```python
from build123d import *

# Parameters (mm, degrees)
SKETCH1_W           = 70
SKETCH1_H           = 40
BOSS_EXTRUDE1_DEPTH = 6.35
SKETCH2_R           = 12.5
SKETCH2_R_2         = 2
CUT_EXTRUDE1_DEPTH  = 81.872260386


with BuildPart() as part:
    # Sketch1 → Boss-Extrude1 (new body)
    with BuildSketch(Plane(origin=(0, 0, 0), x_dir=(1, 0, 0), z_dir=(0, 1, 0))):
        with Locations((35, 20)):
            Rectangle(SKETCH1_W, SKETCH1_H)
    extrude(amount=BOSS_EXTRUDE1_DEPTH)

    # Sketch2 → Cut-Extrude1 (cut, through all)
    with BuildSketch(Plane(origin=(0, 6.35, 0), x_dir=(1, 0, 0), z_dir=(0, 1, 0))):
        with Locations(Location((49.5, 20, 0), (0, 0, 270))):
            Circle(SKETCH2_R)
        with Locations(Location((34, 35.5, 0), (0, 0, 270))):
            Circle(SKETCH2_R_2)
        with Locations(Location((65, 35.5, 0), (0, 0, 270))):
            Circle(SKETCH2_R_2)
        with Locations(Location((65, 4.5, 0), (0, 0, 270))):
            Circle(SKETCH2_R_2)
        with Locations(Location((34, 4.5, 0), (0, 0, 270))):
            Circle(SKETCH2_R_2)
        with BuildLine():
            Line((10, 25), (0, 25))
            Line((0, 25), (0, 15))
            Line((0, 15), (10, 15))
            ThreePointArc((10, 15), (15, 20), (10, 25))
        make_face()
        with BuildLine():
            Line((13, 28), (7, 28))
            ThreePointArc((7, 28), (5, 30), (7, 32))
            Line((7, 32), (13, 32))
            ThreePointArc((13, 32), (15, 30), (13, 28))
        make_face()
        with BuildLine():
            Line((7, 12), (13, 12))
            ThreePointArc((13, 12), (15, 10), (13, 8))
            Line((13, 8), (7, 8))
            ThreePointArc((7, 8), (5, 10), (7, 12))
        make_face()
    extrude(amount=-CUT_EXTRUDE1_DEPTH, mode=Mode.SUBTRACT)


solid = part.part
```
Geometry: final body of the model. Coordinates: model frame, mm. A direction names the side the tool comes from. Round coordinates to 2 decimals unless told otherwise and drop trailing zeros. Write each loop counter-clockwise with the first axis right and the second up, starting at its lowest first coordinate (ties: lowest second). Pieces come first, ordered by that corner, then holes.
Item 1: Section query D-D (z = -22.5). Return loops of the section in (x, y), plus the area to 3 significant figures.
Item 2: Set-up query: faces 5 (the face through (5, 3, -15)), 6 (the face through (35, 6.35, -20)), 7 (the face through (10, 3, -32)). Return all of +Z, -Z, +X, -X, +Y, -Y with unobstructed straight access to the full face (end or side cutting, diameter ignored); none if empty.
Item 3: Pin query (flat end, axial travel): P1, Ø20, axis at x = 49.5, z = -20, coming from the +Y side. Return the tip coordinate at first contact, or that it passes through.
Item 4: Section query B-B (x = 34). Return loops of the section in (y, z).
Item 5: Mould query, pull axis X, two halves, no side actions, for faces 1 (the face through (35, 3, 0)), 2 (the face through (15, 3, -20)), 3 (the face through (15, 3, -30)), 4 (the face through (10, 3, -12)). Classes: +X half, -X half, draft (parallel to the pull), parting line (faces both ways), or undercut.
Item 6: Section query A-A (z = -30). Return loops of the section in (x, y).
Item 7: Section query C-C (y = 4.5). Return loops of the section in (x, z).
Item 8: Material intervals for L1, parallel to X at y = 3.25, z = -4.5; L2, parallel to X at y = 1, z = -9.5; L3, parallel to Z at x = 8.5, y = 2.5, sorted ascending.
Completed:
1. outline: (14.33, 0) - (37.25, 0) - (37.25, 6.35) - (14.33, 6.35) - close; (61.75, 0) - (70, 0) - (70, 6.35) - (61.75, 6.35) - close
1. area: 198 mm2
2. face 5: -X, +Y, -Y
2. face 6: +Z, -Z, +X, -X, +Y
2. face 7: +Y, -Y
3. P1: passes through
4. outline: (0, -40) - (6.35, -40) - (6.35, -37.5) - (0, -37.5) - close; (0, -33.5) - (6.35, -33.5) - (6.35, -6.5) - (0, -6.5) - close; (0, -2.5) - (6.35, -2.5) - (6.35, 0) - (0, 0) - close
5. face 1: draft
5. face 2: -X half
5. face 3: undercut
5. face 4: undercut
6. outline: (0, 0) - (5, 0) - (5, 6.35) - (0, 6.35) - close; (15, 0) - (42, 0) - (42, 6.35) - (15, 6.35) - close; (57, 0) - (70, 0) - (70, 6.35) - (57, 6.35) - close
7. outline: (0, -40) - (70, -40) - (70, 0) - (0, 0) - (0, -15) - (10, -15) arc R5 cw to (10, -25) - (0, -25) - close; hole (7, -32) - (13, -32) arc R2 ccw to (13, -28) - (7, -28) arc R2 ccw to start; hole (7, -12) - (13, -12) arc R2 ccw to (13, -8) - (7, -8) arc R2 ccw to start; hole circle Ø4 at (34, -35.5); hole circle Ø4 at (34, -4.5); hole circle Ø25 at (49.5, -20); hole circle Ø4 at (65, -35.5); hole circle Ø4 at (65, -4.5)
8. L1: x = 0 to 32, 36 to 63, 67 to 70
8. L2: x = 0 to 5.06, 14.94 to 42.72, 56.28 to 70
8. L3: z = -40 to -32, -28 to -25, -15 to -12, -8 to 0
